Source: CAD feature listing. Evaluate the final solid. Frame: model axes, mm. A direction names the side the tool comes from. Coordinates: 2 decimals unless noted, no trailing zeros. Write each loop counter-clockwise with the first axis right and the second up, starting at its lowest first coordinate (ties: lowest second). Pieces come first, ordered by that corner, then holes. Notation, with made-up numbers: (-7, 72.5) -> (51, 72.5) arc R19 ccw to (51, 84.5) -> close; hole circle Ø8 at (-22, 52.25). An arc over 180 degrees is marked (long way). Write item = value, one per line.
from build123d import *

# Parameters (mm, degrees)
F0_R     = 1.6
F0_W     = 21.5
F0_H     = 12.55
F0_W_2   = 16.5
F0_H_2   = 7.55
F1_DEPTH = 1.5
F2_DEPTH = 6.5
F3_W     = 21.5
F3_H     = 12.55
F3_W_2   = 16.5
F3_H_2   = 7.55
F3_W_3   = 14.9
F3_H_3   = 5.95
F4_DEPTH = 1


with BuildPart() as f1:
    # F0 (on Top) → F1 (new body)
    with BuildSketch(Plane.XY):
        with BuildLine():
            Line((-14.25, -9.775), (17.75, -9.775))
            Line((17.75, -9.775), (19.75, -9.775))
            ThreePointArc((19.75, -9.775), (22.5784271247, -8.6034271247), (23.75, -5.775))
            Line((23.75, -5.775), (23.75, 25.325))
            ThreePointArc((23.75, 25.325), (22.5784271247, 28.1534271247), (19.75, 29.325))
            Line((19.75, 29.325), (17.75, 29.325))
            Line((17.75, 29.325), (-14.25, 29.325))
            Line((-14.25, 29.325), (-46.25, 29.325))
            Line((-46.25, 29.325), (-48.25, 29.325))
            ThreePointArc((-48.25, 29.325), (-51.0784271247, 28.1534271247), (-52.25, 25.325))
            Line((-52.25, 25.325), (-52.25, -5.775))
            ThreePointArc((-52.25, -5.775), (-51.0784271247, -8.6034271247), (-48.25, -9.775))
            Line((-48.25, -9.775), (-46.25, -9.775))
            Line((-46.25, -9.775), (-14.25, -9.775))
        make_face()
        with Locations((-46.25, 0)):
            Circle(F0_R, mode=Mode.SUBTRACT)
        with Locations((-28.5, 0)):
            Rectangle(F0_W, F0_H, mode=Mode.SUBTRACT)
        Rectangle(F0_W, F0_H, mode=Mode.SUBTRACT)
        with Locations((17.75, 0)):
            Circle(F0_R, mode=Mode.SUBTRACT)
        with Locations((-46.25, 19.55)):
            Circle(F0_R, mode=Mode.SUBTRACT)
        with Locations((-28.5, 19.55)):
            Rectangle(F0_W, F0_H, mode=Mode.SUBTRACT)
        with Locations((0, 19.55)):
            Rectangle(F0_W, F0_H, mode=Mode.SUBTRACT)
        with Locations((17.75, 19.55)):
            Circle(F0_R, mode=Mode.SUBTRACT)
        with Locations((-28.5, 0)):
            Rectangle(F0_W, F0_H)
        with Locations((-28.5, 0)):
            Rectangle(F0_W_2, F0_H_2, mode=Mode.SUBTRACT)
        Rectangle(F0_W, F0_H)
        Rectangle(F0_W_2, F0_H_2, mode=Mode.SUBTRACT)
        with Locations((-28.5, 19.55)):
            Rectangle(F0_W, F0_H)
        with Locations((-28.5, 19.55)):
            Rectangle(F0_W_2, F0_H_2, mode=Mode.SUBTRACT)
        with Locations((0, 19.55)):
            Rectangle(F0_W, F0_H)
        with Locations((0, 19.55)):
            Rectangle(F0_W_2, F0_H_2, mode=Mode.SUBTRACT)
    extrude(amount=-F1_DEPTH)

    # F0 (on Top) → F2 (join)
    with BuildSketch(Plane.XY):
        Rectangle(F0_W, F0_H)
        Rectangle(F0_W_2, F0_H_2, mode=Mode.SUBTRACT)
        with Locations((-28.5, 0)):
            Rectangle(F0_W, F0_H)
        with Locations((-28.5, 0)):
            Rectangle(F0_W_2, F0_H_2, mode=Mode.SUBTRACT)
        with Locations((-28.5, 19.55)):
            Rectangle(F0_W, F0_H)
        with Locations((-28.5, 19.55)):
            Rectangle(F0_W_2, F0_H_2, mode=Mode.SUBTRACT)
        with Locations((0, 19.55)):
            Rectangle(F0_W, F0_H)
        with Locations((0, 19.55)):
            Rectangle(F0_W_2, F0_H_2, mode=Mode.SUBTRACT)
    extrude(amount=F2_DEPTH)

    # F3 (on face) → F4 (join)
    with BuildSketch(Plane.XY.offset(6.5)):
        with Locations((-28.5, 0)):
            Rectangle(F3_W, F3_H)
        with Locations((-28.5, 0)):
            Rectangle(F3_W_2, F3_H_2, mode=Mode.SUBTRACT)
        Rectangle(F3_W, F3_H)
        Rectangle(F3_W_2, F3_H_2, mode=Mode.SUBTRACT)
        with Locations((-28.5, 19.55)):
            Rectangle(F3_W, F3_H)
        with Locations((-28.5, 19.55)):
            Rectangle(F3_W_2, F3_H_2, mode=Mode.SUBTRACT)
        with Locations((0, 19.55)):
            Rectangle(F3_W, F3_H)
        with Locations((0, 19.55)):
            Rectangle(F3_W_2, F3_H_2, mode=Mode.SUBTRACT)
        with Locations((-28.5, 0)):
            Rectangle(F3_W_2, F3_H_2)
        with Locations((-28.5, 0)):
            Rectangle(F3_W_3, F3_H_3, mode=Mode.SUBTRACT)
        Rectangle(F3_W_2, F3_H_2)
        Rectangle(F3_W_3, F3_H_3, mode=Mode.SUBTRACT)
        with Locations((-28.5, 19.55)):
            Rectangle(F3_W_2, F3_H_2)
        with Locations((-28.5, 19.55)):
            Rectangle(F3_W_3, F3_H_3, mode=Mode.SUBTRACT)
        with Locations((0, 19.55)):
            Rectangle(F3_W_2, F3_H_2)
        with Locations((0, 19.55)):
            Rectangle(F3_W_3, F3_H_3, mode=Mode.SUBTRACT)
    extrude(amount=F4_DEPTH)


solid = f1.part
1) Cut plane A-A, the plane x = 17.75. Output: boundary loops of the cut face in (y, z) (3 decimals).
Answer block:
outline = (-9.775, -1.5) -> (-1.6, -1.5) -> (-1.6, 0) -> (-9.775, 0) -> close; (1.6, -1.5) -> (17.95, -1.5) -> (17.95, 0) -> (1.6, 0) -> close; (21.15, -1.5) -> (29.325, -1.5) -> (29.325, 0) -> (21.15, 0) -> close
2) Material intervals for probe 1 along Y at (x, z) = (-21.5, 4.25) (3 decimals); probe 2 along X at (y, z) = (23, 1.25); probe 3 along Y at (x, z) = (17.75, -0.7) (3 decimals), sorted ascending. Write a range as [from, to].
Answer block:
probe_1 = [-6.275, -3.775], [3.775, 6.275], [13.275, 15.775], [23.325, 25.825]
probe_2 = [-39.25, -36.75], [-20.25, -17.75], [-10.75, -8.25], [8.25, 10.75]
probe_3 = [-9.775, -1.6], [1.6, 17.95], [21.15, 29.325]
3) Reachability of faces 1 (the flat face through (10.75, 19, 4)), 2 (the flat face through (-29, -6.275, 4)), 3 (the flat face through (-39.25, 19, 4)), 4 (the flat face through (-29, 16, 6.5)) from +Z, -Z, +X, -X, +Y, -Y: full face, straight path, thin tool, end or side. Return the list, or none.
Answer block:
face_1 = +Z, +X, +Y, -Y
face_2 = +Z, +X, -X, -Y
face_3 = +Z, -X, +Y, -Y
face_4 = -Z
4) First-contact query: pin 1 Ø2.5 at (x, y) = (-46.25, 19.55) entering from +Z; pin 2 Ø0.5 at (y, z) = (-1, 7) entering from -X; pin 3 Ø2 at (x, z) = (3.5, 3.5) entering from -Y (3 decimals); pin 4 Ø2 at (x, z) = (1, 2.5) entering from +Y (3 decimals). Flat tips, straight axial feed; report the tip coordinate or a pass-through.
Answer block:
pin_1 = through
pin_2 = -39.25
pin_3 = -6.275
pin_4 = 25.825
5) Cut plane D-D, the plane x = -37.5. Output: boundary loops of the cut face in (y, z) (3 decimals), and give its area (3 significant figures).
Answer block:
outline = (-9.775, -1.5) -> (29.325, -1.5) -> (29.325, 0) -> (25.825, 0) -> (25.825, 7.5) -> (13.275, 7.5) -> (13.275, 0) -> (6.275, 0) -> (6.275, 7.5) -> (-6.275, 7.5) -> (-6.275, 0) -> (-9.775, 0) -> close
area = 247 mm2
6) Pull-direction query (X, two-part tool) for faces 5 (the cylindrical face through (-51.11, -8.57, -0.74)), 6 (the flat face through (8.25, 0, 2)), 7 (the flat face through (-29, 15, 7.5)); classes: +X half, -X half, draft (parallel to the pull), parting line (faces both ways), or undercut.
Answer block:
face_5 = -X half
face_6 = undercut
face_7 = draft
7) Cut plane B-B, the plane z = 3.75. Give the number of separate pieces and of enclosed holes in the cut face, and give its area (3 significant figures).
Answer block:
separate_pieces = 4
enclosed_holes = 4
area = 581 mm2
